Check sheet for the modelled part. Datum: model origin and axes. Units: mm. A direction names the side the tool comes from. Round coordinates to 2 decimals unless told otherwise and drop trailing zeros. Order: outer loops, then holes, each group sorted by start corner. A loop starts at its lowest first (then second) coordinate and runs counter-clockwise, first axis right, second up.
(1) Sectioned sample at C-C, the plane x = -10. Enter the section's corners in (y, z), and give its area (3 significant figures).
(2) Depth check by flat-ended pin: pin 1 (5 mm diameter, centred on y = 3.5, z = -3, fed in from -X); pin 2 (12 mm diameter, centred on x = -6, z = -18.5, fed in from -Y); pin 3 (3.5 mm diameter, centred on x = -25, y = 76.5, fed in from +Z); pin 4 (0.9 mm diameter, centred on y = 71, z = -25, fed in from +X). Enter the tip coordinate at first touch or a pass-through.
(3) Sectioned sample at A-A, the plane z = 0. Enter the section's corners in (x, y).
(4) Sectioned sample at B-B, the plane y = 73. Enter the section's corners in (x, z), and give its area (3 significant figures).
(5) Mould release check, pull along X, two halves, no side actions. Record for faces 1 (the flat face through (-12, 130, -6)), 2 (the cylindrical face through (-25, 64, -24)), 3 (the cylindrical face through (-18, 64.2, 18.1)): released by +X, released by -X, zero draft, split by the parting line, or undercut.
(6) Sectioned sample at D-D, the plane z = 19. Enter the section's corners in (x, y).
(7) Tool access check on faces 4 (the cylindrical face through (3.755, 125.07, 11.923)), 5 (the flat face through (21, 5, 8.5)), 6 (the flat face through (-25, 64, 16)), 7 (the cylindrical face through (10.07, 4.93, 20.5)). Record the directions out of +Z, -Z, +X, -X, +Y, -Y that give a thin tool (end or side, any length) a straight path to the whole face; none if there is none.
(8) Thickness scan on probe 1 along X at (y, z) = (4.5, -19); probe 2 along X at (y, z) = (124.5, -15.5); probe 3 along Y at (x, z) = (9, 15.5). Record the ranges inside material, lowest first.
```python
from build123d import *

# Parameters (mm, degrees)
SKETCH1_W           = 52
SKETCH1_H           = 52
BOSS_EXTRUDE1_DEPTH = 10
SKETCH2_W           = 10
SKETCH2_H           = 10
BOSS_EXTRUDE2_DEPTH = 110
SKETCH3_W           = 52
SKETCH3_H           = 52
BOSS_EXTRUDE3_DEPTH = 10
SKETCH4_R           = 12.5
CUT_EXTRUDE1_DEPTH  = 10
SKETCH5_R           = 7.5
CUT_EXTRUDE2_DEPTH  = 10
SKETCH6_W           = 10
SKETCH6_H           = 17
CUT_EXTRUDE3_DEPTH  = 10
SKETCH7_R           = 1.5
CUT_EXTRUDE4_DEPTH  = 10
FILLET1_R           = 5
FILLET2_R           = 2
SKETCH8_R           = 1.5
CUT_EXTRUDE6_DEPTH  = 10
FILLET4_R           = 7


with BuildPart() as part:
    # Sketch1 → Boss-Extrude1 (new body)
    with BuildSketch(Plane(origin=(0, 0, 0), x_dir=(1, 0, 0), z_dir=(0, 1, 0))):
        Rectangle(SKETCH1_W, SKETCH1_H)
    extrude(amount=BOSS_EXTRUDE1_DEPTH)

    # Sketch2 → Boss-Extrude2 (add)
    with BuildSketch(Plane(origin=(0, 10, 0), x_dir=(1, 0, 0), z_dir=(0, 1, 0))):
        with Locations((-21, 21)):
            Rectangle(SKETCH2_W, SKETCH2_H)
        with Locations((21, 21)):
            Rectangle(SKETCH2_W, SKETCH2_H)
        with Locations((-21, -21)):
            Rectangle(SKETCH2_W, SKETCH2_H)
        with Locations((21, -21)):
            Rectangle(SKETCH2_W, SKETCH2_H)
    extrude(amount=BOSS_EXTRUDE2_DEPTH)

    # Sketch3 → Boss-Extrude3 (add)
    with BuildSketch(Plane(origin=(0, 120, 0), x_dir=(1, 0, 0), z_dir=(0, 1, 0))):
        Rectangle(SKETCH3_W, SKETCH3_H)
    extrude(amount=BOSS_EXTRUDE3_DEPTH)

    # Sketch4 → Cut-Extrude1 (cut)
    with BuildSketch(Plane(origin=(0, 130, 0), x_dir=(1, 0, 0), z_dir=(0, 1, 0))):
        with Locations(Location((0, 0, 0), (0, 0, 270))):
            Circle(SKETCH4_R)
    extrude(amount=-CUT_EXTRUDE1_DEPTH, mode=Mode.SUBTRACT)

    # Sketch5 → Cut-Extrude2 (cut)
    with BuildSketch(Plane.XZ):
        with Locations(Location((0, 0, 0), (0, 0, 270))):
            Circle(SKETCH5_R)
    extrude(amount=-CUT_EXTRUDE2_DEPTH, mode=Mode.SUBTRACT)

    # Sketch6 → Cut-Extrude3 (cut)
    with BuildSketch(Plane.XZ):
        with Locations((-21, 0)):
            Rectangle(SKETCH6_W, SKETCH6_H)
        with Locations((21, 0)):
            Rectangle(SKETCH6_W, SKETCH6_H)
    extrude(amount=-CUT_EXTRUDE3_DEPTH, mode=Mode.SUBTRACT)

    # Sketch7 → Cut-Extrude4 (cut)
    with BuildSketch(Plane.XZ):
        with Locations(Location((10, 19, 0), (0, 0, 270))):
            Circle(SKETCH7_R)
        with Locations(Location((-10, 19, 0), (0, 0, 90))):
            Circle(SKETCH7_R)
        with Locations(Location((10, -19, 0), (0, 0, 90))):
            Circle(SKETCH7_R)
        with Locations(Location((-10, -19, 0), (0, 0, 270))):
            Circle(SKETCH7_R)
    extrude(amount=-CUT_EXTRUDE4_DEPTH, mode=Mode.SUBTRACT)

    # Fillet1
    fillet1_edges = [part.edges().sort_by_distance(p)[0] for p in [
        (26, 65, 26),
        (-26, 65, 26),
        (-26, 65, -26),
        (26, 65, -26),
    ]]
    fillet(fillet1_edges, radius=FILLET1_R)

    # Fillet2
    fillet2_edges = [part.edges().sort_by_distance(p)[0] for p in [
        (-16, 5, -8.5),
        (-16, 5, 8.5),
        (-26, 5, 8.5),
        (-26, 5, -8.5),
        (16, 5, 8.5),
        (16, 5, -8.5),
        (26, 5, -8.5),
        (26, 5, 8.5),
    ]]
    fillet(fillet2_edges, radius=FILLET2_R)

    # Sketch8 → Cut-Extrude6 (cut)
    with BuildSketch(Plane(origin=(0, 130, 0), x_dir=(1, 0, 0), z_dir=(0, 1, 0))):
        with Locations(Location((-15.5, -15.5, 0), (0, 0, 270))):
            Circle(SKETCH8_R)
        with Locations(Location((-15.5, 15.5, 0), (0, 0, 270))):
            Circle(SKETCH8_R)
        with Locations(Location((15.5, 15.5, 0), (0, 0, 270))):
            Circle(SKETCH8_R)
        with Locations(Location((15.5, -15.5, 0), (0, 0, 270))):
            Circle(SKETCH8_R)
    extrude(amount=-CUT_EXTRUDE6_DEPTH, mode=Mode.SUBTRACT)

    # Fillet4
    # the kernel refuses this fillet: 7 mm, written as the material it takes off along each edge
    with BuildSketch(Plane(origin=(-16, 10, -16), x_dir=(-1, 0, 0), z_dir=(0, 1, 0)), Plane(origin=(16, 10, -16), x_dir=(0, 0, -1), z_dir=(0, 1, 0)), Plane(origin=(16, 10, 16), x_dir=(1, 0, 0), z_dir=(0, 1, 0))) as fillet4_piece_1:
        with BuildLine():
            CenterArc((FILLET4_R, -FILLET4_R), FILLET4_R, 90, 90)
            Line((0, -FILLET4_R), (0, 0))
            Line((0, 0), (FILLET4_R, 0))
        make_face()
    extrude(amount=110, mode=Mode.SUBTRACT)
    with BuildSketch(Plane(origin=(-16, 10, 16), x_dir=(-1, 0, 0), z_dir=(0, 1, 0))) as fillet4_piece_2:
        with BuildLine():
            CenterArc((FILLET4_R, FILLET4_R), FILLET4_R, 180, 90)
            Line((0, FILLET4_R), (0, 0))
            Line((0, 0), (FILLET4_R, 0))
        make_face()
    extrude(amount=110, mode=Mode.SUBTRACT)


solid = part.part
```
Derived:
1. outline: (0, -26) - (10, -26) - (10, -20.5) - (0, -20.5) - close; (0, -17.5) - (10, -17.5) - (10, 17.5) - (0, 17.5) - close; (0, 20.5) - (10, 20.5) - (10, 26) - (0, 26) - close; (120, -26) - (130, -26) - (130, -7.5) - (120, -7.5) - close; (120, 7.5) - (130, 7.5) - (130, 26) - (120, 26) - close
1. area: 830 mm2
2. pin 1: stops at x = -16
2. pin 2: stops at y = 0
2. pin 3: stops at z = 25.47
2. pin 4: stops at x = 24.52
3. outline: (-26, 120) - (-12.5, 120) - (-12.5, 130) - (-26, 130) - close; (-16, 0) - (-7.5, 0) - (-7.5, 10) - (-16, 10) - close; (7.5, 0) - (16, 0) - (16, 10) - (7.5, 10) - close; (12.5, 120) - (26, 120) - (26, 130) - (12.5, 130) - close
4. outline: (-26, -21) arc R5 ccw to (-21, -26) - (-16, -26) - (-16, -23) arc R7 ccw to (-23, -16) - (-26, -16) - close; (-26, 16) - (-23, 16) arc R7 ccw to (-16, 23) - (-16, 26) - (-21, 26) arc R5 ccw to (-26, 21) - close; (16, -26) - (21, -26) arc R5 ccw to (26, -21) - (26, -16) - (23, -16) arc R7 ccw to (16, -23) - close; (16, 23) arc R7 ccw to (23, 16) - (26, 16) - (26, 21) arc R5 ccw to (21, 26) - (16, 26) - close
4. area: 336 mm2
5. face 1: zero draft
5. face 2: released by -X
5. face 3: undercut
6. outline: (-26, 0) - (-11.5, 0) - (-11.5, 10) - (-17.26, 10) - (-17.26, 120) - (17.26, 120) - (17.26, 10) - (11.5, 10) - (11.5, 0) - (26, 0) - (26, 130) - (-26, 130) - close; (-8.5, 0) - (8.5, 0) - (8.5, 10) - (-8.5, 10) - close
7. face 4: +Y
7. face 5: +X, -Y
7. face 6: +X, -X
7. face 7: -Y
8. probe 1: x = -26 to -11.5, -8.5 to 8.5, 11.5 to 26
8. probe 2: x = -26 to -17, -14 to 14, 17 to 26
8. probe 3: y = 0 to 10, 120 to 130
